Build history of the part. All positions in model axes, mm. Give positions to 0.01 mm unless a question says otherwise; leave off trailing zeros. Order: outer loops, then holes, each group sorted by start corner. A loop starts at its lowest first (then second) coordinate and runs counter-clockwise, first axis right, second up. Notation, with made-up numbers: (49, -18.5) - (54, -18.5) arc R20 ccw to (54, -12.5) - close; hole circle Ø5 at (88.5, -21). An arc over 180 degrees is marked (long way). Use a Markdown table: item, result.
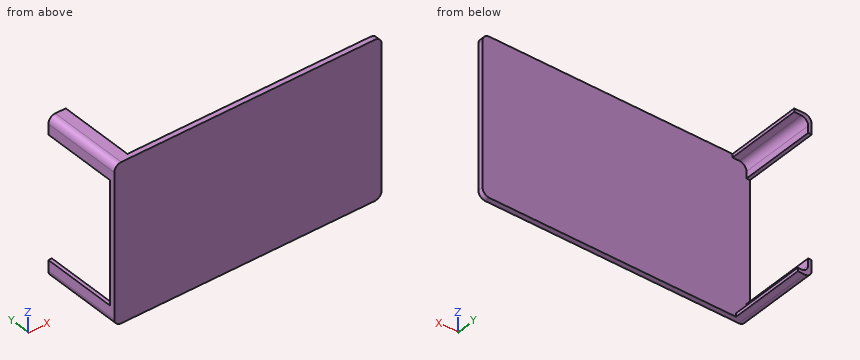
from build123d import *

# Parameters (mm, degrees)
EXTRUDE_1_DEPTH     = 23.5
SKETCH_3_3_W        = 1
SKETCH_3_3_H        = 35
SKETCH_3_3_W_2      = 69
SKETCH_3_3_H_2      = 1
SKETCH_3_3_W_3      = 67
SKETCH_3_3_H_3      = 37
EXTRUDE_2_DEPTH     = 1.5
SKETCH_6_W          = 1
SKETCH_6_H          = 37
SKETCH_6_H_2        = 35
SKETCH_6_W_2        = 67
SKETCH_6_H_3        = 1
SKETCH_6_W_3        = 69
CUT_EXTRUDE_1_DEPTH = 22
CUT_EXTRUDE_START   = -22
CUT_EXTRUDE_2_DEPTH = 22


with BuildPart() as part:
    # Sketch 3 → Extrude 1 (new body)
    with BuildSketch(Plane(origin=(0, 0, 0), x_dir=(1, 0, 0), z_dir=(0, 1, 0))):
        with BuildLine():
            Line((-36, 16), (37, 16))
            ThreePointArc((37, 16), (38.414213562, 15.414213562), (39, 14))
            Line((39, 14), (39, -27))
            ThreePointArc((39, -27), (38.414213562, -28.414213562), (37, -29))
            Line((37, -29), (-36, -29))
            ThreePointArc((-36, -29), (-37.414213562, -28.414213562), (-38, -27))
            Line((-38, -27), (-38, 14))
            ThreePointArc((-38, 14), (-37.414213562, 15.414213562), (-36, 16))
        make_face()
        with BuildLine():
            Line((-35, -28), (36, -28))
            ThreePointArc((36, -28), (37.414213562, -27.414213562), (38, -26))
            Line((38, -26), (38, 13))
            ThreePointArc((38, 13), (37.414213562, 14.414213562), (36, 15))
            Line((36, 15), (-35, 15))
            ThreePointArc((-35, 15), (-36.414213562, 14.414213562), (-37, 13))
            Line((-37, 13), (-37, -26))
            ThreePointArc((-37, -26), (-36.414213562, -27.414213562), (-35, -28))
        make_face(mode=Mode.SUBTRACT)
    extrude(amount=EXTRUDE_1_DEPTH)

    # Sketch 3_3 → Extrude 2 (add)
    with BuildSketch(Plane(origin=(0, 0, 0), x_dir=(1, 0, 0), z_dir=(0, 1, 0))):
        with BuildLine():
            Line((-37, -26), (-37, 13))
            ThreePointArc((-37, 13), (-36.414213562, 14.414213562), (-35, 15))
            Line((-35, 15), (36, 15))
            ThreePointArc((36, 15), (37.414213562, 14.414213562), (38, 13))
            Line((38, 13), (38, -26))
            ThreePointArc((38, -26), (37.414213562, -27.414213562), (36, -28))
            Line((36, -28), (-35, -28))
            ThreePointArc((-35, -28), (-36.414213562, -27.414213562), (-37, -26))
        make_face()
        with Locations((-37.5, -6.5)):
            Rectangle(SKETCH_3_3_W, SKETCH_3_3_H)
        with Locations((0.5, 15.5)):
            Rectangle(SKETCH_3_3_W_2, SKETCH_3_3_H_2)
        with Locations((0.5, -28.5)):
            Rectangle(SKETCH_3_3_W_3, SKETCH_3_3_H_2)
        with Locations((38.5, -6.5)):
            Rectangle(SKETCH_3_3_W, SKETCH_3_3_H_3)
    extrude(amount=EXTRUDE_2_DEPTH)

    # Sketch 6 → Cut-Extrude 1 (cut)
    with BuildSketch(Plane(origin=(0, 23.5, 0), x_dir=(1, 0, 0), z_dir=(0, 1, 0))):
        with Locations((38.5, -6.5)):
            Rectangle(SKETCH_6_W, SKETCH_6_H)
        with Locations((-37.5, -6.5)):
            Rectangle(SKETCH_6_W, SKETCH_6_H_2)
        with Locations((0.5, -28.5)):
            Rectangle(SKETCH_6_W_2, SKETCH_6_H_3)
        with Locations((0.5, 15.5)):
            Rectangle(SKETCH_6_W_3, SKETCH_6_H_3)
    extrude(amount=-CUT_EXTRUDE_1_DEPTH, mode=Mode.SUBTRACT)

    # Sketch 9 → Cut-Extrude 2 (cut)
    with BuildSketch(Plane(origin=(0, 23.5, 0), x_dir=(1, 0, 0), z_dir=(0, 1, 0)).offset(CUT_EXTRUDE_START)):
        with BuildLine():
            Line((38, 12), (39, 12))
            Line((39, 12), (39, 14))
            ThreePointArc((39, 14), (38.414213562, 15.414213562), (37, 16))
            Line((37, 16), (35, 16))
            Line((35, 16), (35, 15))
            Line((35, 15), (36, 15))
            ThreePointArc((36, 15), (37.414213562, 14.414213562), (38, 13))
            Line((38, 13), (38, 12))
        make_face()
        with BuildLine():
            Line((39, -27), (39, -25))
            Line((39, -25), (38, -25))
            Line((38, -25), (38, -26))
            ThreePointArc((38, -26), (37.414213562, -27.414213562), (36, -28))
            Line((36, -28), (34, -28))
            Line((34, -28), (34, -29))
            Line((34, -29), (37, -29))
            ThreePointArc((37, -29), (38.414213562, -28.414213562), (39, -27))
        make_face()
    extrude(amount=CUT_EXTRUDE_2_DEPTH, mode=Mode.SUBTRACT)


solid = part.part
1) Slice it at A-A (y = 17.5). Write the cut outline in (x, z).
Computed:
| item | result |
|---|---|
| outline | (-38, -14) arc R2 ccw to (-36, -16) - (-34, -16) - (-34, -15) - (-35, -15) arc R2 cw to (-37, -13) - (-37, -11) - (-38, -11) - close; (-38, 24) - (-37, 24) - (-37, 26) arc R2 cw to (-35, 28) - (-33, 28) - (-33, 29) - (-36, 29) arc R2 ccw to (-38, 27) - close |
2) Wall check: line 1 (Y direction, x = -34.5, z = -7); line 2 (X direction, y = 2.5, z = 27); line 3 (X direction, y = 16, z = 26.5). Give the ranges that are in metal, low to high. Write a range as from..to.
Computed:
| item | result |
|---|---|
| line 1 | y = 0..1.5 |
| line 2 | x = -38..-36.73 |
| line 3 | x = -38..-36.94 |
3) Slice it at B-B (x = -24.5). Write the cut outline in (y, z), and give its area (3 significant figures).
Computed:
| item | result |
|---|---|
| outline | (0, -16) - (1.5, -16) - (1.5, 29) - (0, 29) - close |
| area | 67.5 mm² |
4) Slice it at C-C (z = 16). Write the cut outline in (x, y), and give its area (4 significant figures).
Computed:
| item | result |
|---|---|
| outline | (-38, 0) - (39, 0) - (39, 1.5) - (-38, 1.5) - close |
| area | 115.5 mm² |
5) Pin check, flat tips, straight feed: P1, Ø8, axis at y = 7, z = 22, coming from the +X side; P2, Ø0.8, axis at x = -37.5, y = 13, coming from the +Z side; P3, Ø1.1, axis at y = 10.5, z = 28.5, coming from the +X side. Stop position of each tip, or through.
Computed:
| item | result |
|---|---|
| P1 | stops at x = -37 |
| P2 | stops at z = 28.67 |
| P3 | stops at x = -33 |
